Check sheet for the modelled part. Datum: model origin and axes. Units: mm. Face numbers are marked on the shaded views. A direction names the side the tool comes from. Coordinates: 2 decimals unless noted, no trailing zeros. Write each loop counter-clockwise with the first axis right and the second up, starting at its lowest first coordinate (ties: lowest second). Pieces come first, ordered by that corner, then holes. Notation, with made-up numbers: (47, 24.5) - (77, 24.5) arc R18 cw to (77, 30.5) - close; hole circle Ø6 at (66.25, -4). An arc over 180 degrees is marked (long way). Use one line per item in the form item = value. Start each with the question number.
1. Tool access check on the marked faces 5, 6 and 7. Record the directions out of +Z, -Z, +X, -X, +Y, -Y that give a thin tool (end or side, any length) a straight path to the whole face; none if there is none.
2. Cross-section at D-D on x = 13.5. Record the boundary of the cut face in (y, z).
3. Cross-section at B-B on z = -7. Record the boundary of the cut face in (x, y).
4. Go/stop test with flat-tipped pins: pin 1 Ø5 at (x, y) = (-9, 19.5) entering from -Z; pin 2 Ø4 at (x, z) = (20, -3.5) entering from +Y; pin 3 Ø1 at (y, z) = (12.5, -7.5) entering from -X. Record where each tip stops, or that it passes through.
5. Cross-section at C-C on y = 20. Record the boundary of the cut face in (x, z), then the cut area to 3 significant figures.
6. Draft check along Z on the marked faces 1, 2, 3 and 4. Enter one of: +Z half, -Z half, draft (parallel to the pull), parting line (faces both ways), or undercut.
7. Scan lines: line 1 along Y through (x, z) = (0, -8.95); line 2 along Y through (x, z) = (-15, -1.5); line 3 along Z through (x, y) = (-18, 10). Record each from-to range of solid material in increasing order.
8. Cross-section at A-A on x = 0. Record the boundary of the cut face in (y, z), then the cut area to 3 significant figures.
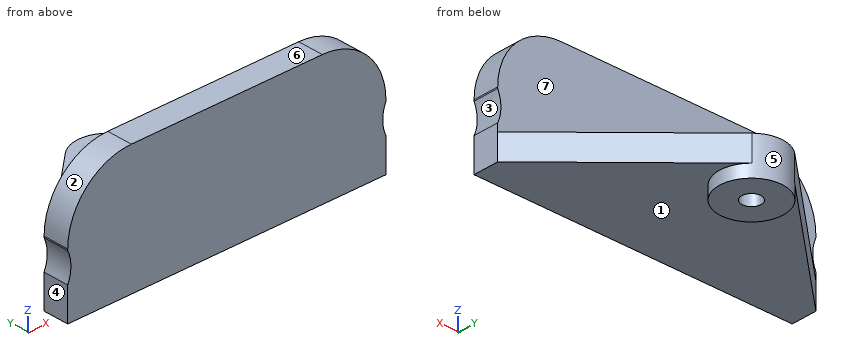
```python
from build123d import *

# Parameters (mm, degrees)
CROQUIS1_W              = 50
CROQUIS1_H              = 20
SALIENTE_EXTRUIR1_DEPTH = 4
CROQUIS2_R              = 5
CROQUIS2_R_2            = 1.5
SALIENTE_EXTRUIR4_DEPTH = 4
SALIENTE_EXTRUIR5_START = 2
CROQUIS2_3_R            = 5
CROQUIS2_3_R_2          = 1.5
SALIENTE_EXTRUIR5_DEPTH = 2
CORTAR_EXTRUIR1_REACH   = 36.785
CROQUIS5_R              = 5.5
REDONDEO1_R             = 10


with BuildPart() as part:
    # Croquis1 → Saliente-Extruir1 (new body)
    with BuildSketch(Plane(origin=(0, 0, 0), x_dir=(1, 0, 0), z_dir=(0, 1, 0))):
        Rectangle(CROQUIS1_W, CROQUIS1_H)
    extrude(amount=SALIENTE_EXTRUIR1_DEPTH)

    # Croquis2 → Saliente-Extruir4 (add)
    # profile 1 of 2: a face of its own
    with BuildSketch(Plane(origin=(0, 0, -10), x_dir=(-1, 0, 0), z_dir=(0, 0, -1))):
        with BuildLine():
            Line((-3.366172774, 23.69714496), (-25, 4))
            Line((-25, 4), (25, 4))
            Line((25, 4), (3.366172774, 23.69714496))
            ThreePointArc((3.366172774, 23.69714496), (4.573339254, 22.021031436), (5, 20))
            ThreePointArc((5, 20), (-2.021031436, 15.426660746), (-3.366172774, 23.69714496))
        make_face()
    # profile 2 of 2: a face of its own
    with BuildSketch(Plane(origin=(0, 0, -10), x_dir=(-1, 0, 0), z_dir=(0, 0, -1))):
        with Locations((0, 20)):
            Circle(CROQUIS2_R)
        with Locations((0, 20)):
            Circle(CROQUIS2_R_2, mode=Mode.SUBTRACT)
    extrude(amount=-SALIENTE_EXTRUIR4_DEPTH)

    # Croquis2_3 → Saliente-Extruir5 (add)
    with BuildSketch(Plane(origin=(0, 0, -10), x_dir=(-1, 0, 0), z_dir=(0, 0, -1)).offset(SALIENTE_EXTRUIR5_START)):
        with Locations((0, 20)):
            Circle(CROQUIS2_3_R)
        with Locations((0, 20)):
            Circle(CROQUIS2_3_R_2, mode=Mode.SUBTRACT)
    extrude(amount=-SALIENTE_EXTRUIR5_DEPTH)

    # Croquis5 → Cortar-Extruir1 (cut, up to next)
    with BuildSketch(Plane(origin=(0, 4, 0), x_dir=(1, 0, 0), z_dir=(0, 1, 0)), mode=Mode.PRIVATE) as cortar_extruir1_sk1:
        with Locations((-30, 2.5)):
            Circle(CROQUIS5_R)
    cortar_extruir1_tool1 = extrude(cortar_extruir1_sk1.sketch, amount=-CORTAR_EXTRUIR1_REACH, mode=Mode.PRIVATE) & part.part
    # Croquis5 → Cortar-Extruir1 (cut, up to next)
    with BuildSketch(Plane(origin=(0, 4, 0), x_dir=(1, 0, 0), z_dir=(0, 1, 0)), mode=Mode.PRIVATE) as cortar_extruir1_sk2:
        with Locations((30, 2.5)):
            Circle(CROQUIS5_R)
    cortar_extruir1_tool2 = extrude(cortar_extruir1_sk2.sketch, amount=-CORTAR_EXTRUIR1_REACH, mode=Mode.PRIVATE) & part.part
    add(cortar_extruir1_tool1.solids().sort_by_distance((-30, 4, -2.5))[0], mode=Mode.SUBTRACT)
    add(cortar_extruir1_tool2.solids().sort_by_distance((30, 4, -2.5))[0], mode=Mode.SUBTRACT)

    # Redondeo1
    redondeo1_edges = [part.edges().sort_by_distance(p)[0] for p in [
        (25, 2, 10),
        (-25, 2, 10),
    ]]
    fillet(redondeo1_edges, radius=REDONDEO1_R)


solid = part.part
```
Final values:
q1.face_5 = -Z
q1.face_6 = +Z, +X, -X, +Y, -Y
q1.face_7 = +Z, +X, -X, +Y
q2.outline = (0, -10) - (14.47, -10) - (14.47, -6) - (4, -6) - (4, 10) - (0, 10) - close
q3.outline = (-25, 0) - (25, 0) - (25, 4) - (3.37, 23.7) arc R5 ccw to (-3.37, 23.7) - (-25, 4) - close; hole circle Ø3 at (0, 20)
q4.pin_1 = -10
q4.pin_2 = 4
q4.pin_3 = -16.21
q5.outline = (-7.43, -10) - (-5, -10) - (-5, -12) - (-1.5, -12) - (-1.5, -6) - (-7.43, -6) - close; (1.5, -12) - (5, -12) - (5, -10) - (7.43, -10) - (7.43, -6) - (1.5, -6) - close
q5.area = 61.4 mm²
q6.face_1 = -Z half
q6.face_2 = +Z half
q6.face_3 = undercut
q6.face_4 = draft
q7.line_1 = 0 to 18.5, 21.5 to 25
q7.line_2 = 0 to 4
q7.line_3 = -10 to -6
q8.outline = (0, -10) - (15, -10) - (15, -12) - (18.5, -12) - (18.5, -6) - (4, -6) - (4, 10) - (0, 10) - close; (21.5, -12) - (25, -12) - (25, -6) - (21.5, -6) - close
q8.area = 166 mm²
